Input: dimensioned drawing with shaded views. Units: mm. Origin: part minimum x, y, z. A direction names the side the tool comes from. Coordinates: 2 decimals unless noted, no trailing zeros. Order: outer loops, then holes, each group sorted by start corner. A loop starts at its lowest first (then second) coordinate and runs counter-clockwise, first axis right, second up. Notation, with made-up numbers: (25, 83.25) - (50, 83.25) arc R14 ccw to (50, 109.25) - close; hole circle Ø4 at (7.5, -13.5). An arc over 180 degrees is marked (long way). One line per question, with ' | ' between items. Start each with the question number.
(1) Section C-C (y = 1). Return the cut outline in (x, z).
(2) Section A-A (z = 3.5). Return the cut outline in (x, y).
(3) Contact query for flat-ended pins moving along their axis: P1, Ø1.5, axis at x = 26.5, z = 3, coming from the +Y side; P2, Ø2, axis at y = 6.5, z = 7.5, coming from the +X side; P3, Ø5, axis at y = 8, z = 5, coming from the +X side. Output: stop coordinate, or through.
(4) Draft query along X for the marked faces 1, 2, 3 and 4. Return one class per face: +X half, -X half, draft (parallel to the pull), parting line (faces both ways), or undercut.
(5) Access query for the marked faces 5 and 6. Directions: +Z, -Z, +X, -X, +Y, -Y. A direction counts if a zero-diameter tool reaches every point of the face in a straight line with its end or side. Return the directions, or none.
(6) Section B-B (y = 9.5). Return the cut outline in (x, z).
(7) Line query: line 1 along X through (y, z) = (18.5, 5.75); line 2 along X through (y, z) = (8.25, 3.5); line 3 along Y through (x, z) = (23.5, 2). Output: solid intervals per line, ascending.
(8) Section D-D (x = 21.5). Return the cut outline in (y, z), then the cut area to 3 significant figures.
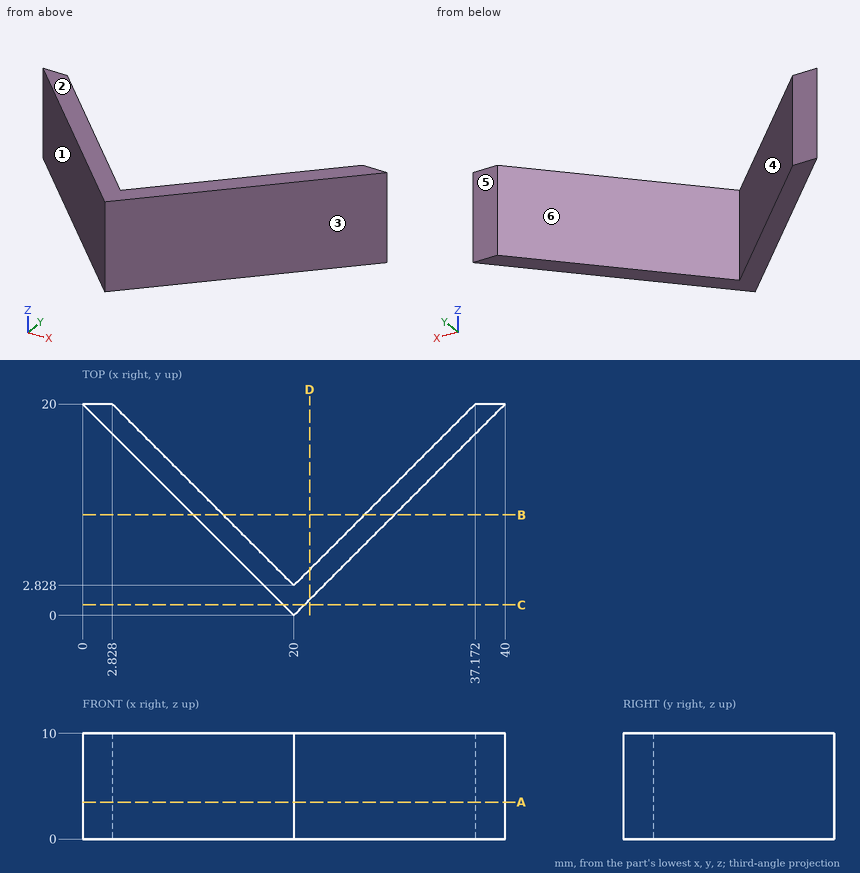
Response values:
1) outline: (19, 0) - (21, 0) - (21, 10) - (19, 10) - close
2) outline: (0, 20) - (20, 0) - (40, 20) - (37.17, 20) - (20, 2.83) - (2.83, 20) - close
3) P1: stops at y = 10.08 | P2: stops at x = 27.5 | P3: stops at x = 30.5
4) face 1: -X half | face 2: draft | face 3: +X half | face 4: undercut
5) face 5: +Z, -Z, +X, -X, +Y | face 6: +Z, -Z, +Y
6) outline: (10.5, 0) - (13.33, 0) - (13.33, 10) - (10.5, 10) - close; (26.67, 0) - (29.5, 0) - (29.5, 10) - (26.67, 10) - close
7) line 1: x = 1.5 to 4.33, 35.67 to 38.5 | line 2: x = 11.75 to 14.58, 25.42 to 28.25 | line 3: y = 3.5 to 6.33
8) outline: (1.5, 0) - (4.33, 0) - (4.33, 10) - (1.5, 10) - close | area: 28.3 mm²
